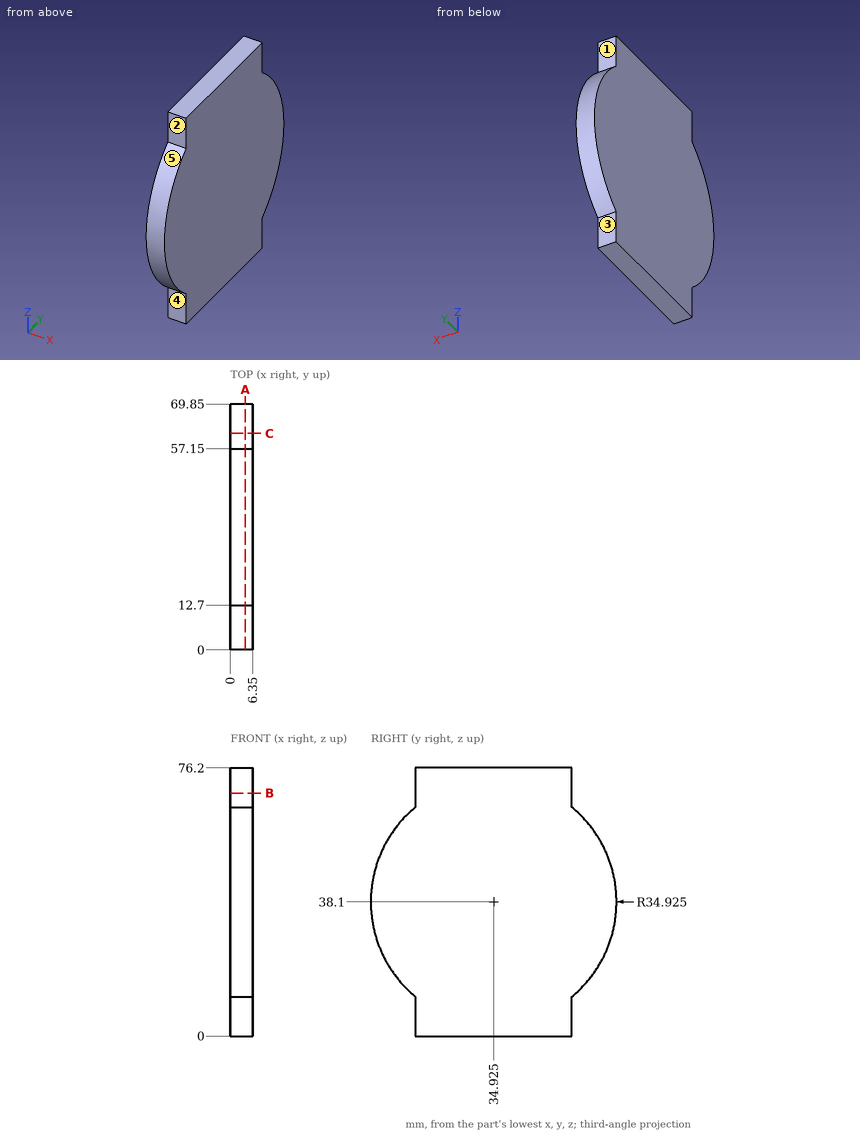
Here's the drawing with two shaded views (mm, measured from the low corner). I have some questions. A direction names the side the tool comes from. Give positions to 0.01 mm unless a question says otherwise; leave off trailing zeros. Loops run counter-clockwise (first coordinate to the right, second up) from the corner with the lowest first, then second, coordinate; pieces in that order, holes last. Notation, with made-up numbers: M -22,60.5 L 37,60.5 A27 cw 37,82.5 Z; hole C 75,-2.75 d1. An arc over 180 degrees is marked long. Use one line per item in the form item = value. Start each with the question number.
Q1. If we section it at B-B (z = 69): Write out the boundary of the cut face in (x, y), then the cut area to 3 significant figures.
Q2. If we section it at A-A (x = 4.25): Write out the boundary of the cut face in (y, z) (3 decimals), then the cut area to 3 significant figures.
Q3. I need wall thicknesses on line 1 along Y through (x, z) = (3.25, 70); line 2 along Z through (x, y) = (3.75, 8.5); line 3 along Y through (x, z) = (4.75, 49). Which ranges of each line are inside material? Lowest first, please.
Q4. Which directions (+Z, -Z, +X, -X, +Y, -Y) give clear straight access to the entire face, cutting with the end or side of a thin tool? Please do the marked faces 1, 2, 3, 4 and 5.
Q5. If we section it at C-C (y = 61.5): Write out the boundary of the cut face in (x, z), then the cut area to 3 significant figures.
Q6. Will these pins go through, and if not, where does the flat tip stop? pin 1 Ø1.9 at (x, z) = (3, 6) entering from -Y; pin 2 Ø1.9 at (x, z) = (1.5, 73) entering from +Y; pin 3 Ø3 at (x, z) = (0.5, 45.5) entering from +Y.
Taken from the geometry:
q1.outline = M 0,12.7 L 6.35,12.7 L 6.35,57.15 L 0,57.15 Z
q1.area = 282 mm^2
q2.outline = M 12.7,0 L 57.15,0 L 57.15,11.159 A34.925 ccw 57.15,65.041 L 57.15,76.2 L 12.7,76.2 L 12.7,65.041 A34.925 ccw 12.7,11.159 Z
q2.area = 4,340 mm^2
q3.line_1 = 12.7 to 57.15
q3.line_2 = 15.26 to 60.94
q3.line_3 = 1.74 to 68.11
q4.face_1 = +Z, +X, -X, +Y
q4.face_2 = +Z, +X, -X, -Y
q4.face_3 = -Z, +X, -X, +Y
q4.face_4 = -Z, +X, -X, -Y
q4.face_5 = +X, -X, -Y
q5.outline = M 0,15.44 L 6.35,15.44 L 6.35,60.76 L 0,60.76 Z
q5.area = 288 mm^2
q6.pin_1 = 12.7
q6.pin_2 = 57.15
q6.pin_3 = 69.35
